```python
from build123d import *

# Parameters (mm, degrees)
PAD_DEPTH       = 20
SKETCH004_R     = 2
POCKET002_DEPTH = 142.001
SKETCH005_R     = 2
POCKET003_DEPTH = 85.001


with BuildPart() as part:
    # Sketch → Pad (new body)
    with BuildSketch(Plane.XY):
        Polygon((-10, -42.5), (132, -42.5), (132, -30.5), (0, -30.5), (0, 30.5), (132, 30.5), (132, 42.5), (-10, 42.5), (-10, 38.5), (-17, 38.5), (-17, 33.5), (-10, 33.5), (-10, -33.5), (-17, -33.5), (-17, -38.5), (-10, -38.5), align=None)
    extrude(amount=PAD_DEPTH)

    # Sketch004 → Pocket002 (cut, through all)
    with BuildSketch(Plane(origin=(-10, 0, 0), x_dir=(0, -1, 0), z_dir=(-1, 0, 0))):
        with Locations((0, 10)):
            Circle(SKETCH004_R)
    extrude(amount=-POCKET002_DEPTH, mode=Mode.SUBTRACT)

    # Sketch005 → Pocket003 (cut, through all)
    with BuildSketch(Plane.XZ.offset(42.5)):
        with Locations((-5, 10)):
            Circle(SKETCH005_R)
        with Locations((122, 10)):
            Circle(SKETCH005_R)
    extrude(amount=-POCKET003_DEPTH, mode=Mode.SUBTRACT)


solid = part.part
```
CAD build for the part. Positions are in the model's coordinates, mm. A direction names the side the tool comes from. Round coordinates to 2 decimals unless told otherwise and drop trailing zeros. Order: outer loops, then holes, each group sorted by start corner. A loop starts at its lowest first (then second) coordinate and runs counter-clockwise, first axis right, second up.
Item 1: Saw through at B-B on y = -22.5. Write the cut outline in (x, z).
Item 2: Mould opens along Z. For faces 1 (the face through (-5, -22, 12)), 2 (the face through (52, 32, 0)), 3 (the face through (52, 32, 20)), 4 (the face through (-10, -40, 10)) say: pulls with the +Z half, pulls with the -Z half, needs draft (parallel to the pull), parting line crosses it, or undercut.
Item 3: Pin check, flat tips, straight feed: pin 1 (3 mm diameter, centred on y = 19, z = 7, fed in from -X); pin 2 (2 mm diameter, centred on x = -15, z = 14, fed in from +Y); pin 3 (6.5 mm diameter, centred on y = 0, z = 10, fed in from +X). Stop position of each tip, or through.
Item 4: Tool access for faces 5 (the face through (0, -0.4, 7.6)), 6 (the face through (-13, -33.5, 10)), 7 (the face through (-17, -36, 10)), 8 (the face through (-14, -38.5, 10)), 9 (the face through (-13, 38.5, 10)): list every direction of +Z, -Z, +X, -X, +Y, -Y with a clear straight run to the whole face (end or side of a thin tool).
Item 5: Probe line 1 along Y through (x, z) = (-11, 14.5); line 2 along Y through (x, z) = (58, 1); line 3 along X through (y, z) = (-27.5, 10). List the from-to ranges inside material, lowest first.
Item 6: Saw through at C-C on z = 4.5. Write the cut outline in (x, y), then the cut area to 3 significant figures.
Item 7: Saw through at A-A on x = 114.5. Write the cut outline in (y, z).
Reported:
1. outline: (-10, 0) - (0, 0) - (0, 20) - (-10, 20) - close; hole circle Ø4 at (-5, 10)
2. face 1: undercut
2. face 2: pulls with the -Z half
2. face 3: pulls with the +Z half
2. face 4: needs draft
3. pin 1: stops at x = -10
3. pin 2: stops at y = 38.5
3. pin 3: stops at x = 0
4. face 5: +Z, -Z, +X
4. face 6: +Z, -Z, -X
4. face 7: +Z, -Z, -X, +Y, -Y
4. face 8: +Z, -Z, -X, -Y
4. face 9: +Z, -Z, -X, +Y
5. line 1: y = -38.5 to -33.5, 33.5 to 38.5
5. line 2: y = -42.5 to -30.5, 30.5 to 42.5
5. line 3: x = -10 to -7, -3 to 0
6. outline: (-17, -38.5) - (-10, -38.5) - (-10, -42.5) - (132, -42.5) - (132, -30.5) - (0, -30.5) - (0, 30.5) - (132, 30.5) - (132, 42.5) - (-10, 42.5) - (-10, 38.5) - (-17, 38.5) - (-17, 33.5) - (-10, 33.5) - (-10, -33.5) - (-17, -33.5) - close
6. area: 4,090 mm2
7. outline: (-42.5, 0) - (-30.5, 0) - (-30.5, 20) - (-42.5, 20) - close; (30.5, 0) - (42.5, 0) - (42.5, 20) - (30.5, 20) - close
